```python
from build123d import *

# Parameters (mm, degrees)
SKIZZE1_W                       = 155
SKIZZE1_H                       = 140
SKIZZE1_W_2                     = 127
SKIZZE1_H_2                     = 112
AUFSATZ_LINEAR_AUSTRAGEN1_DEPTH = 10
SKIZZE2_W                       = 14
SKIZZE2_H                       = 14
AUFSATZ_LINEAR_AUSTRAGEN2_DEPTH = 60
SKIZZE3_R                       = 5
AUFSATZ_LINEAR_AUSTRAGEN3_DEPTH = 10
VERRUNDUNG1_R                   = 5
VERRUNDUNG3_R                   = 45
VERRUNDUNG4_R                   = 45
VERRUNDUNG6_R                   = 45
VERRUNDUNG7_R                   = 45
AUFSATZ_LINEAR_START            = 5
SKIZZE9_R                       = 5
AUFSATZ_LINEAR_AUSTRAGEN4_DEPTH = 5
VERRUNDUNG8_R                   = 5


# Some blends are built 0.0001 mm under size
with BuildPart() as part:
    # Skizze1 → Aufsatz-Linear austragen1 (new body)
    with BuildSketch(Plane.XY):
        Rectangle(SKIZZE1_W, SKIZZE1_H)
        Rectangle(SKIZZE1_W_2, SKIZZE1_H_2, mode=Mode.SUBTRACT)
    extrude(amount=AUFSATZ_LINEAR_AUSTRAGEN1_DEPTH)

    # Skizze2 → Aufsatz-Linear austragen2 (add)
    with BuildSketch(Plane.XY.offset(10)):
        with Locations((-70.5, 63)):
            Rectangle(SKIZZE2_W, SKIZZE2_H)
        with Locations((70.5, 63)):
            Rectangle(SKIZZE2_W, SKIZZE2_H)
        with Locations((70.5, -63)):
            Rectangle(SKIZZE2_W, SKIZZE2_H)
        with Locations((-70.5, -63)):
            Rectangle(SKIZZE2_W, SKIZZE2_H)
    extrude(amount=AUFSATZ_LINEAR_AUSTRAGEN2_DEPTH)

    # Skizze3 → Aufsatz-Linear austragen3 (add)
    with BuildSketch(Plane.XY.offset(70)):
        with Locations(Location((-70.5, -62.673227844, 0), (0, 0, 180))):
            Circle(SKIZZE3_R)
        with Locations((70.5, -62.673227844)):
            Circle(SKIZZE3_R)
        with Locations(Location((70.5, 63, 0), (0, 0, 180))):
            Circle(SKIZZE3_R)
        with Locations((-70.5, 63)):
            Circle(SKIZZE3_R)
    extrude(amount=AUFSATZ_LINEAR_AUSTRAGEN3_DEPTH)

    # Verrundung1
    verrundung1_edges = [part.edges().sort_by_distance(p)[0] for p in [
        (-65.5, -62.673227844, 80),
        (65.5, -62.673227844, 80),
        (75.5, 63, 80),
        (-75.5, 63, 80),
    ]]
    fillet(verrundung1_edges, radius=VERRUNDUNG1_R)

    # Verrundung3
    # the kernel refuses this fillet: 45 mm, written as the material it adds along each edge
    with BuildSketch(Plane(origin=(-63.5, -70, 10), x_dir=(0, 0, 1), z_dir=(0, 1, 0))) as verrundung3_piece_1:
        with BuildLine():
            CenterArc((VERRUNDUNG3_R, VERRUNDUNG3_R), VERRUNDUNG3_R, 180, 90)
            Line((0, VERRUNDUNG3_R), (0, 0))
            Line((0, 0), (VERRUNDUNG3_R, 0))
        make_face()
    extrude(amount=14)

    # Verrundung4
    verrundung4_edges = [part.edges().sort_by_distance(p)[0] for p in [
        (-70.5, -56, 10),
    ]]
    fillet(verrundung4_edges, radius=VERRUNDUNG4_R - 0.0001)  # a hair under: the kernel refuses the full size

    # Verrundung6
    # the kernel refuses this fillet: 45 mm, written as the material it adds along each edge
    with BuildSketch(Plane(origin=(-63.5, 70, 10), x_dir=(0, 0, 1), z_dir=(0, -1, 0)), Plane(origin=(63.5, 70, 10), x_dir=(-1, 0, 0), z_dir=(0, -1, 0)), Plane(origin=(63.5, -70, 10), x_dir=(0, 0, 1), z_dir=(0, 1, 0))) as verrundung6_piece_1:
        with BuildLine():
            CenterArc((VERRUNDUNG6_R, -VERRUNDUNG6_R), VERRUNDUNG6_R, 90, 90)
            Line((0, -VERRUNDUNG6_R), (0, 0))
            Line((0, 0), (VERRUNDUNG6_R, 0))
        make_face()
    extrude(amount=14)
    with BuildSketch(Plane(origin=(-63.5, 70, 10), x_dir=(0, 0, 1), z_dir=(0, -1, 0))) as verrundung6_piece_2_section:
        with BuildLine():
            CenterArc((VERRUNDUNG6_R, -VERRUNDUNG6_R), VERRUNDUNG6_R, 90, 90)
            Line((0, -VERRUNDUNG6_R), (0, 0))
            Line((0, 0), (VERRUNDUNG6_R, 0))
        make_face()
    verrundung6_piece_2 = extrude(amount=126.5, mode=Mode.PRIVATE)
    verrundung6_piece_2 = split(verrundung6_piece_2, bisect_by=Plane(origin=(-53.312219858, -56, 20.187780141), z_dir=(0, -1, 0)), keep=Keep.TOP, mode=Mode.PRIVATE)
    add(verrundung6_piece_2)
    with BuildSketch(Plane(origin=(63.5, 70, 10), x_dir=(-1, 0, 0), z_dir=(0, -1, 0))) as verrundung6_piece_3_section:
        with BuildLine():
            CenterArc((VERRUNDUNG6_R, -VERRUNDUNG6_R), VERRUNDUNG6_R, 90, 90)
            Line((0, -VERRUNDUNG6_R), (0, 0))
            Line((0, 0), (VERRUNDUNG6_R, 0))
        make_face()
    verrundung6_piece_3 = extrude(amount=126.5, mode=Mode.PRIVATE)
    verrundung6_piece_3 = split(verrundung6_piece_3, bisect_by=Plane(origin=(53.312219858, -56, 20.187780142), z_dir=(0, -1, 0)), keep=Keep.TOP, mode=Mode.PRIVATE)
    add(verrundung6_piece_3)
    with BuildSketch(Plane(origin=(63.5, -70, 10), x_dir=(0, 0, 1), z_dir=(0, 1, 0))) as verrundung6_piece_4_section:
        with BuildLine():
            CenterArc((VERRUNDUNG6_R, -VERRUNDUNG6_R), VERRUNDUNG6_R, 90, 90)
            Line((0, -VERRUNDUNG6_R), (0, 0))
            Line((0, 0), (VERRUNDUNG6_R, 0))
        make_face()
    verrundung6_piece_4 = extrude(amount=126.5, mode=Mode.PRIVATE)
    verrundung6_piece_4 = split(verrundung6_piece_4, bisect_by=Plane(origin=(53.312219858, 56, 20.187780142), z_dir=(0, 1, 0)), keep=Keep.TOP, mode=Mode.PRIVATE)
    add(verrundung6_piece_4)

    # Verrundung7
    verrundung7_edges = [part.edges().sort_by_distance(p)[0] for p in [
        (-70.5, 56, 10),
        (70.5, 56, 10),
        (70.5, -56, 10),
    ]]
    fillet(verrundung7_edges, radius=VERRUNDUNG7_R)

    # Skizze9 → Aufsatz-Linear austragen4 (add)
    with BuildSketch(Plane(origin=(0, 0, 0), x_dir=(-1, 0, 0), z_dir=(0, 0, -1)).offset(AUFSATZ_LINEAR_START)):
        with Locations((70.5, -62.673227844)):
            Circle(SKIZZE9_R)
        with Locations((70.5, 63)):
            Circle(SKIZZE9_R)
        with Locations((-70.5, 63)):
            Circle(SKIZZE9_R)
        with Locations((-70.5, -62.673227844)):
            Circle(SKIZZE9_R)
    extrude(amount=-AUFSATZ_LINEAR_AUSTRAGEN4_DEPTH)

    # Verrundung8
    verrundung8_edges = [part.edges().sort_by_distance(p)[0] for p in [
        (-65.5, -62.673227844, -5),
        (-65.5, 63, -5),
        (75.5, 63, -5),
        (75.5, -62.673227844, -5),
    ]]
    fillet(verrundung8_edges, radius=VERRUNDUNG8_R - 0.0001)  # a hair under: the kernel refuses the full size


solid = part.part
```
Geometry check sheet. Reference: the model listing, model coordinates, mm. A direction names the side the tool comes from. Coordinates: 2 decimals unless noted, no trailing zeros. Write each loop counter-clockwise with the first axis right and the second up, starting at its lowest first coordinate (ties: lowest second). Pieces come first, ordered by that corner, then holes. Notation, with made-up numbers: M 66,72.25 L 89,72.25 A18 cw 89,98.25 Z; hole C -15,0 d5. An arc over 180 degrees is marked long. Use one line per item in the form item = value. Start each with the question number.
1) Thickness scan on probe 1 along X at (y, z) = (58, 63); probe 2 along Y at (x, z) = (62, 33); probe 3 along Y at (x, z) = (-67.5, 16). Record the ranges inside material, lowest first. Write a range as from..to.
2) Go/stop test with flat-tipped pins: pin 1 Ø4 at (x, y) = (5.5, -66.5) entering from +Z; pin 2 Ø15.5 at (x, y) = (-71.5, 5.5) entering from +Z; pin 3 Ø10 at (x, z) = (46, 27.5) entering from -Y. Record where each tip stops, or that it passes through.
3) Release check for a two-part mould opening along Y. For faces 1 (the flat face through (-63.5, 0, 5)), 2 (the cylindrical face through (49.968, 63.098, 22.832)), 3 (the flat face through (-1, 70, 4)), 4 (the flat face through (-72, 68, 70)) record: pulls with the +Y half, pulls with the -Y half, needs draft (parallel to the pull), parting line crosses it, or undercut.
4) Set-up check for faces 5 (the cylindrical face through (70.598, 43.168, 23.532)), 6 (the cylindrical face through (50.668, -63.098, 23.532)), 7 (the flat face through (69, -68, 70)), 8 (the flat face through (63.5, 0, 5)): record each of +Z, -Z, +X, -X, +Y, -Y from which the full face is reachable in a straight line by a thin tool's end or side.
5) Section check B-B on z = 4. Enter the section's corners in (x, y).
6) Section check D-D on z = 40.5. State how many separate pieces and enclosed holes the cut face has, and give its area (3 significant figures).
7) Section check A-A on x = -13. Enter the section's corners in (y, z).
8) Section check C-C on y = 21. Enter the section's corners in (x, z), and give its area (3 significant figures).
Responses:
q1.probe_1 = -77.5..-63.5, 63.5..77.5
q1.probe_2 = -70..-56, 56..70
q1.probe_3 = -70..-33.45, 33.45..70
q2.pin_1 = 10
q2.pin_2 = 10.06
q2.pin_3 = through
q3.face_1 = undercut
q3.face_2 = needs draft
q3.face_3 = pulls with the +Y half
q3.face_4 = undercut
q4.face_5 = +Z, +X, -X
q4.face_6 = +Z, +Y, -Y
q4.face_7 = +Z
q4.face_8 = +Z, -Z
q5.outline = M -77.5,-70 L 77.5,-70 L 77.5,70 L -77.5,70 Z; hole M -63.5,-56 L 63.5,-56 L 63.5,56 L -63.5,56 Z
q6.separate_pieces = 4
q6.enclosed_holes = 0
q6.area = 1,050 mm2
q7.outline = M -70,0 L -56,0 L -56,10 L -70,10 Z; M 56,0 L 70,0 L 70,10 L 56,10 Z
q8.outline = M -77.5,0 L -63.5,0 L -63.5,11.13 L -77.5,11.13 Z; M 63.5,0 L 77.5,0 L 77.5,11.13 L 63.5,11.13 Z
q8.area = 312 mm2
